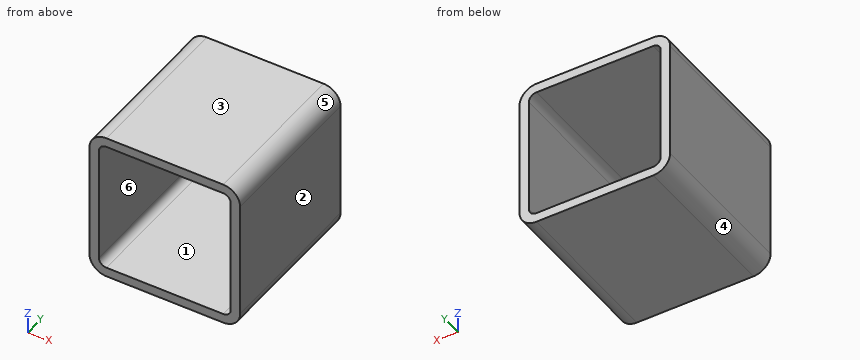
Solid Edge part; units mm, degrees
sketch "Sketch1" plane through (0, 0, 0) normal (1, 0, 0) x (0, 1, 0)
  line L0 (0, 0) -> (53.8724, 0)
sketch "Sketch2" plane through (0, 0, 0) normal (0, -1, 0) x (1, 0, 0)
  line L0 (25.4, -19.685) -> (25.4, 19.685)
  arc A0 (19.685, 25.4) -> (25.4, 19.685) centre (19.685, 19.685) cw
  line L1 (19.685, 25.4) -> (-19.685, 25.4)
  arc A1 (-19.685, 25.4) -> (-25.4, 19.685) centre (-19.685, 19.685) ccw
  line L2 (-25.4, 19.685) -> (-25.4, -19.685)
  arc A2 (-25.4, -19.685) -> (-19.685, -25.4) centre (-19.685, -19.685) ccw
  line L3 (-19.685, -25.4) -> (19.685, -25.4)
  arc A3 (19.685, -25.4) -> (25.4, -19.685) centre (19.685, -19.685) ccw
sweep "Protrusion_1" add profiles "Sketch2" path "Sketch1"
sketch "Sketch3" plane through (0, 0, 0) normal (1, 0, 0) x (0, 1, 0)
  line L0 (0, 0) -> (53.8724, 0)
sketch "Sketch4" plane through (0, 0, 0) normal (0, -1, 0) x (1, 0, 0)
  line L0 (-19.685, -22.225) -> (19.685, -22.225)
  arc A0 (19.685, -22.225) -> (22.225, -19.685) centre (19.685, -19.685) ccw
  line L1 (22.225, -19.685) -> (22.225, 19.685)
  arc A1 (22.225, 19.685) -> (19.685, 22.225) centre (19.685, 19.685) ccw
  line L2 (19.685, 22.225) -> (-19.685, 22.225)
  arc A2 (-19.685, 22.225) -> (-22.225, 19.685) centre (-19.685, 19.685) ccw
  line L3 (-22.225, 19.685) -> (-22.225, -19.685)
  arc A3 (-22.225, -19.685) -> (-19.685, -22.225) centre (-19.685, -19.685) ccw
sweep "Cutout_1" cut profiles "Sketch4" path "Sketch3"
Geometry: final body of the model. Coordinates: model frame, mm. Face numbers are marked on the shaded views. A direction names the side the tool comes from. Coordinates: 2 decimals unless noted, no trailing zeros. Write each loop counter-clockwise with the first axis right and the second up, starting at its lowest first coordinate (ties: lowest second). Pieces come first, ordered by that corner, then holes. Notation, with made-up numbers: (-2, 55.5) - (56, 55.5) arc R17 ccw to (56, 77.5) - close; hole circle Ø1 at (11.25, 88.25). An arc over 180 degrees is marked (long way). Return JSON: item names as keys, results as strings.
Item 1: Section query C-C (y = 37). Output: boundary loops of the cut face in (x, z) (3 decimals).
Completed:
{"outline": "(-25.4, -19.685) arc R5.715 ccw to (-19.685, -25.4) - (19.685, -25.4) arc R5.715 ccw to (25.4, -19.685) - (25.4, 19.685) arc R5.715 ccw to (19.685, 25.4) - (-19.685, 25.4) arc R5.715 ccw to (-25.4, 19.685) - close; hole (-22.225, -19.685) arc R2.54 ccw to (-19.685, -22.225) - (19.685, -22.225) arc R2.54 ccw to (22.225, -19.685) - (22.225, 19.685) arc R2.54 ccw to (19.685, 22.225) - (-19.685, 22.225) arc R2.54 ccw to (-22.225, 19.685) - close"}
Item 2: Section query B-B (x = 17). Output: boundary loops of the cut face in (y, z) (3 decimals), and give its area (3 significant figures).
Completed:
{"outline": "(0, -25.4) - (53.872, -25.4) - (53.872, -22.225) - (0, -22.225) - close; (0, 22.225) - (53.872, 22.225) - (53.872, 25.4) - (0, 25.4) - close", "area": "342 mm2"}
Item 3: Pull-direction query (Z, two-part tool) for the marked faces 1, 2, 3 and 4; classes: +Z half, -Z half, draft (parallel to the pull), parting line (faces both ways), or undercut.
Completed:
{"face 1": "undercut", "face 2": "draft", "face 3": "+Z half", "face 4": "-Z half"}
Item 4: Reachability of the marked faces 5 and 6 from +Z, -Z, +X, -X, +Y, -Y: full face, straight path, thin tool, end or side. Return the list, or none.
Completed:
{"face 5": "+Z, +X, +Y, -Y", "face 6": "+Y, -Y"}
Item 5: Section query A-A (z = -7). Output: boundary loops of the cut face in (x, y) (3 decimals), and give its area (3 significant figures).
Completed:
{"outline": "(-25.4, 0) - (-22.225, 0) - (-22.225, 53.872) - (-25.4, 53.872) - close; (22.225, 0) - (25.4, 0) - (25.4, 53.872) - (22.225, 53.872) - close", "area": "342 mm2"}
Item 6: Line query: L1, parallel to Z at x = -19, y = 14.5 (3 decimals); L2, parallel to X at y = 44, z = 21. Output: solid intervals per line, ascending.
Completed:
{"L1": "z = -25.4 to -22.225, 22.225 to 25.4", "L2": "x = -25.25 to -21.86, 21.86 to 25.25"}
